Can you work these out from the model? Positions are in its coordinate system, mm. Coordinates: 2 decimals unless noted, no trailing zeros. Loops run counter-clockwise (first coordinate to the right, second up) from the corner with the lowest first, then second, coordinate; pieces in that order, holes last. Notation, with made-up numbers: (81, 41.5) -> (110, 41.5) arc R9 cw to (110, 51.5) -> close; hole circle Ø5 at (-2, 27.5). An arc over 180 degrees is marked (long way). Use one line per item in the form item = value. Start each with the question number.
(1) I need wall thicknesses on line 1 (X direction, y = -11, z = -1.4); line 2 (Y direction, x = -70, z = -3); line 3 (X direction, y = -66, z = -0.75). Which ranges of each line are inside material? Lowest first, please. Write a range as [from, to].
(2) Imagine slicing it at B-B (z = -2.55). State how many separate pieces and enclosed holes the cut face has, plus the area to 3 significant figures.
(3) Imagine slicing it at C-C (x = -17.5). List the corners of the cut face in (y, z) for me.
(4) Imagine slicing it at A-A (y = 101.9). List the corners of the cut face in (x, z) for me.
(5) I'm going to push a flat-ended pin straight in: pin 1 (1.5 mm diameter, centred on x = 41, z = -2, fed in from -Y). Where does the tip first touch, or does it pass through?
(6) Thinking about a two-plate mould opening in Y: for faces 1 (the cylindrical face through (-139.72, 98.35, -1.77)), 2 (the flat face through (-6, 17, 0)), 3 (the cylindrical face through (63.54, -128.23, -1.77)), which applies, released by +Y, released by -Y, zero draft, split by the parting line, or undercut?
```python
from build123d import *

# Parameters (mm, degrees)
BASE_FLANGE1_DEPTH    = 3.5
SKETCH2_R             = 3.5
CUT_EXTRUDE1_DEPTH    = 3.5
SKETCH3_R             = 4
CUT_EXTRUDE2_DEPTH    = 3.5
F_8_0MM_DOWEL_HOLE1_D = 8
F_8_0MM_DOWEL_HOLE2_D = 8


# Sheet-metal steps are written as plain solids
with BuildPart() as part:
    # Sketch1 → Base-Flange1 (new body)
    with BuildSketch(Plane.XY):
        Polygon((-54.2366, -134.59778982), (-54.2366, -10.36118982), (45.7634, -10.36118982), (45.7634, -134.59778982), (137.5, -134.59778982), (137.5, 110), (-145.9732, 110), (-145.9732, -134.59778982), align=None)
    extrude(amount=-BASE_FLANGE1_DEPTH)

    # Sketch2 → Cut-Extrude1 (cut)
    with BuildSketch(Plane(origin=(0, 0, -3.5), x_dir=(-1, 0, 0), z_dir=(0, 0, -1))):
        with Locations((-60.7634, -126.09778982)):
            Circle(SKETCH2_R)
        with Locations((69.2366, -126.09778982)):
            Circle(SKETCH2_R)
        with Locations((-60.7634, -63.09778982)):
            Circle(SKETCH2_R)
        with Locations((69.2366, -63.09778982)):
            Circle(SKETCH2_R)
    extrude(amount=-CUT_EXTRUDE1_DEPTH, mode=Mode.SUBTRACT)

    # Sketch3 → Cut-Extrude2 (cut)
    with BuildSketch(Plane(origin=(0, 0, -3.5), x_dir=(-1, 0, 0), z_dir=(0, 0, -1))):
        with Locations((137.8732, 101.9)):
            Circle(SKETCH3_R)
        with Locations((-129.4, 101.9)):
            Circle(SKETCH3_R)
        with Locations((-129.4, -108.47319982)):
            Circle(SKETCH3_R)
        with Locations((137.8732, -108.47319982)):
            Circle(SKETCH3_R)
    extrude(amount=-CUT_EXTRUDE2_DEPTH, mode=Mode.SUBTRACT)

    # Ø8.0mm Dowel Hole1 (through all)
    with Locations(Plane(origin=(-128.31605397, 74.62471448, 0), x_dir=(1, 0, 0), z_dir=(0, 0, 1))):
        with Locations((256.29328213, -53.092411223)):
            Hole(F_8_0MM_DOWEL_HOLE1_D / 2)

    # Ø8.0mm Dowel Hole2 (through all)
    with Locations(Plane(origin=(-128.31605397, 74.62471448, 0), x_dir=(1, 0, 0), z_dir=(0, 0, 1))):
        with Locations((-7.072415731, -53.092411223)):
            Hole(F_8_0MM_DOWEL_HOLE2_D / 2)


solid = part.part
```
Worked out:
q1.line_1 = [-145.97, -54.24], [45.76, 137.5]
q1.line_2 = [-134.6, -129.51], [-122.68, -66.51], [-59.68, 110]
q1.line_3 = [-145.97, -71.19], [-67.28, -54.24], [45.76, 58.81], [62.72, 137.5]
q2.separate_pieces = 1
q2.enclosed_holes = 10
q2.area = 56,500 mm2
q3.outline = (-10.36, -3.5) -> (110, -3.5) -> (110, 0) -> (-10.36, 0) -> close
q4.outline = (-145.97, -3.5) -> (-141.87, -3.5) -> (-141.87, 0) -> (-145.97, 0) -> close; (-133.87, -3.5) -> (125.4, -3.5) -> (125.4, 0) -> (-133.87, 0) -> close; (133.4, -3.5) -> (137.5, -3.5) -> (137.5, 0) -> (133.4, 0) -> close
q5.pin_1 = -10.36
q6.face_1 = undercut
q6.face_2 = zero draft
q6.face_3 = undercut
